Autodesk Inventor part; units mm, degrees
ref_plane "YZ Plane" through (0, 0, 0) normal (1, 0, 0) x (0, 1, 0)
ref_plane "XZ Plane" through (0, 0, 0) normal (0, 1, 0) x (-1, 0, 0)
ref_plane "XY Plane" through (0, 0, 0) normal (0, 0, 1) x (1, 0, 0)
sketch "Sketch1" plane through (0, 0, 0) normal (0, 1, 0) x (-1, 0, 0)
  circle A0 centre (0, 0) radius 20
  dimension "d0" = 40
extrude "Extrusion1" add sketch "Sketch1" along normal blind 10
sketch "Sketch2" plane through (0, 10, 0) normal (0, 1, 0) x (1, 0, 0)
  circle A0 centre (0, 0) radius 20
  circle A1 centre (0, 0) radius 6
  dimension "d3" = 12
extrude "Extrusion2" cut sketch "Sketch2" against normal blind 10 contours A1
sketch "Sketch3" plane through (0, 10, 0) normal (0, 1, 0) x (1, 0, 0)
  circle A0 centre (-12.593, 0) radius 1.5
  circle A1 centre (12.593, 0) radius 1.5
  dimension "d7" = 3
  dimension "d8" = 3
extrude "Extrusion3" cut sketch "Sketch3" against normal blind 10
sketch "Sketch6" plane through (0, 10, 0) normal (0, 1, 0) x (1, 0, 0)
  circle A0 centre (0, 0) radius 6
  circle A1 centre (0, 0) radius 20
  circle A2 centre (0, 0) radius 5
  dimension "d11" = 10
extrude "Extrusion4" add sketch "Sketch6" against normal blind 10 contours A0
sketch "Sketch7" plane through (0, 10, 0) normal (0, 1, 0) x (1, 0, 0)
  circle A0 centre (0, 0) radius 5
  circle A1 centre (0, 0) radius 20
  circle A2 centre (0, 0) radius 3
  dimension "d14" = 6
extrude "Extrusion5" add sketch "Sketch7" against normal blind 2 contours A0
sketch "Sketch8" plane through (0, 10, 0) normal (0, 1, 0) x (1, 0, 0)
  circle A0 centre (0, 0) radius 20
  line L0 (9, 17.8606) -> (9, 7.8606)
  line L1 (9, 7.8606) -> (-9, 7.8606)
  line L2 (-9, 7.8606) -> (-9, 17.8606)
  line L3 (-9, 17.8606) -> (9, 7.8606) construction
  line L4 (9, 17.8606) -> (-9, 7.8606) construction
  arc A1 (9, 17.8606) -> (-9, 17.8606) centre (0, 0) ccw
  point P0 (0, 12.8606)
  dimension "d17" = 18
  dimension "d18" = 10
extrude "Extrusion6" cut sketch "Sketch8" against normal blind 10 contours L0 L1 L2 A0 picked at (0, 11.9071)
sketch "Sketch9" plane through (0, 10, 0) normal (0, 1, 0) x (1, 0, 0)
  line L0 (-9, 7.8606) -> (9, 7.8606)
  line L1 (9, 7.8606) -> (9, 5.8606)
  line L2 (9, 5.8606) -> (-9, 5.8606)
  line L3 (-9, 5.8606) -> (-9, 7.8606)
  dimension "d21" = 18
  dimension "d25" = 2
extrude "Extrusion7" cut sketch "Sketch9" against normal blind 10
sketch "Sketch10" plane through (0, 0, 0) normal (0, -1, 0) x (1, 0, 0)
  circle A0 centre (0, 0) radius 5
extrude "Extrusion8" add sketch "Sketch10" against normal blind 8
sketch "Sketch11" plane through (0, 8, 0) normal (0, 1, 0) x (1, 0, 0)
  circle A0 centre (0, 0) radius 3
extrude "Extrusion9" cut sketch "Sketch11" against normal blind 8
sketch "Sketch12" plane through (0, 10, 0) normal (0, 1, 0) x (1, 0, 0)
  circle A0 centre (0, 0) radius 3
  arc A1 (-9, 17.8606) -> (9, 17.8606) centre (0, 0) ccw
  circle A2 centre (0, 0) radius 2
  dimension "d32" = 4
extrude "Extrusion10" add sketch "Sketch12" against normal blind 10
fillet "Fillet1" radius 1 2 edges at (9, 5, -5.8606) (-9, 5, -5.8606)
properties part number "ruka_lozisko"
Verification items for the finished model (mm, model axes). A direction names the side the tool comes from. Coordinates: 2 decimals unless noted, no trailing zeros. Order: outer loops, then holes, each group sorted by start corner. A loop starts at its lowest first (then second) coordinate and runs counter-clockwise, first axis right, second up. Notation, with made-up numbers: M 16,52 L 28,52 A17 ccw 28,71 Z; hole C -1,-5 d7. An arc over 180 degrees is marked long. One line per item, written item: value. Start each with the question number.
Item 1: Sectioned sample at C-C (y = 3.25). Enter the section's corners in (x, z).
Item 2: Access from +Z, -Z, +X, -X, +Y, -Y to the whole of each face (thin tool, end or side, straight path). Record for faces 1 (the flat face through (0, 5, -5.861)), 2 (the cylindrical face through (0, 5, 2)).
Item 3: Sectioned sample at A-A (x = 0). Enter the section's corners in (y, z).
Item 4: Gauge pin test, flat ends, axial feed: pin 1 (3 mm diameter, centred on x = 13, y = 2.5, fed in from -Z); pin 2 (3 mm diameter, centred on y = 3, z = -12, fed in from +X); pin 3 (1.5 mm diameter, centred on x = 15, y = 8.5, fed in from -Z). Record the tip position at first contact, or that the pin passes through.
Item 5: Sectioned sample at D-D (z = -11.5). Enter the section's corners in (x, y), then the cut area to 3 significant figures.
Item 6: Sectioned sample at B-B (z = 0). Enter the section's corners in (x, y).
Item 7: Mould release check, pull along X, two halves, no side actions. Record for faces 3 (the flat face through (0, 0, 5)), 4 (the cylindrical face through (0.749, 4.93, 19.986)), 5 (the cylindrical face through (8.715, 4.93, -6.161)): released by +X, released by -X, zero draft, split by the parting line, or undercut.
Item 8: Scan lines: probe 1 along X at (y, z) = (7, 0); probe 2 along Z at (x, y) = (0, 5.5); probe 3 along Z at (x, y) = (11.5, 4.5). Record each from-to range of solid material in increasing order.
Conclusion:
1. outline: M -9,-17.86 L -9,-6.86 A1 cw -8,-5.86 L 8,-5.86 A1 cw 9,-6.86 L 9,-17.86 A20 ccw long Z; hole C -12.59,0 d3; hole C 0,0 d4; hole C 12.59,0 d3
2. face 1: -Z, +Y, -Y
2. face 2: +Y, -Y
3. outline: M 0,-5.86 L 10,-5.86 L 10,-2 L 0,-2 Z; M 0,2 L 10,2 L 10,20 L 0,20 Z
4. pin 1: stops at z = -16.36
4. pin 2: stops at x = 17.02
4. pin 3: stops at z = -14.03
5. outline: M -16.36,0 L -9,0 L -9,10 L -16.36,10 Z; M 9,0 L 16.36,0 L 16.36,10 L 9,10 Z
5. area: 147 mm^2
6. outline: M -20,0 L -14.09,0 L -14.09,10 L -20,10 Z; M -11.09,0 L -2,0 L -2,10 L -11.09,10 Z; M 2,0 L 11.09,0 L 11.09,10 L 2,10 Z; M 14.09,0 L 20,0 L 20,10 L 14.09,10 Z
7. face 3: zero draft
7. face 4: split by the parting line
7. face 5: undercut
8. probe 1: x = -20 to -14.09, -11.09 to -2, 2 to 11.09, 14.09 to 20
8. probe 2: z = -5.86 to -2, 2 to 20
8. probe 3: z = -16.36 to -1.03, 1.03 to 16.36
